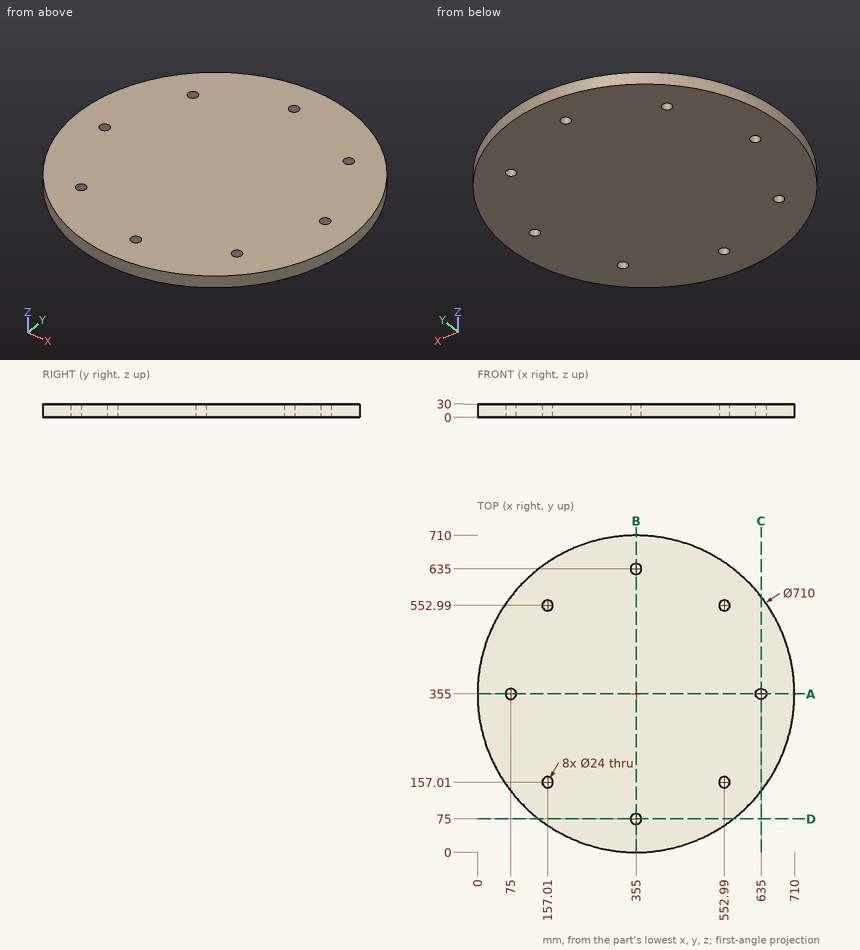
Source: three-view drawing plus pictorial views. Frame: mm from the lowest corner of the part. Round coordinates to 2 decimals unless told otherwise and drop trailing zeros. Order: outer loops, then holes, each group sorted by start corner. A loop starts at its lowest first (then second) coordinate and runs counter-clockwise, first axis right, second up. Notation, with made-up numbers: (89.25, 59) -> (147.25, 59) arc R19 cw to (147.25, 88) -> close; hole circle Ø6 at (83, -18). An arc over 180 degrees is marked (long way). Use CSV: the item, a comma, the result in double quotes. Start each with the question number.
1) Section C-C (x = 635). Return the cut outline in (y, z).
2) Section A-A (y = 355). Return the cut outline in (x, z), and give its area (3 significant figures).
3) First-contact query: pin 1 Ø4 at (y, z) = (397.5, 22) entering from +X; pin 2 Ø6 at (y, z) = (262, 14.5) entering from -X; pin 3 Ø8 at (y, z) = (169.5, 19.5) entering from +X. Flat tips, straight axial feed; report the tip coordinate or a pass-through.
4) Material intervals for line 1 along X through (y, z) = (83.5, 7); line 2 along X through (y, z) = (347, 16.75); line 3 along Y through (x, z) = (635, 9.75), sorted ascending. Write a range as from..to.
Returned:
1,outline,"(136.77, 0) -> (343, 0) -> (343, 30) -> (136.77, 30) -> close; (367, 0) -> (573.23, 0) -> (573.23, 30) -> (367, 30) -> close"
2,outline,"(0, 0) -> (63, 0) -> (63, 30) -> (0, 30) -> close; (87, 0) -> (623, 0) -> (623, 30) -> (87, 30) -> close; (647, 0) -> (710, 0) -> (710, 30) -> (647, 30) -> close"
2,area,"19,900 mm²"
3,pin 1,"stops at x = 707.68"
3,pin 2,"stops at x = 11.6"
3,pin 3,"stops at x = 660.09"
4,line 1,"x = 126.28..346.53, 363.47..583.72"
4,line 2,"x = 0.09..66.06, 83.94..626.06, 643.94..709.91"
4,line 3,"y = 136.77..343, 367..573.23"
